Check sheet for the modelled part. Datum: model origin and axes. Units: mm. Face numbers are marked on the shaded views. A direction names the side the tool comes from. Round coordinates to 2 decimals unless told otherwise and drop trailing zeros. Order: outer loops, then holes, each group sorted by start corner. A loop starts at its lowest first (then second) coordinate and runs counter-clockwise, first axis right, second up.
(1) Tool access check on the marked faces 1 and 2. Record the directions out of +Z, -Z, +X, -X, +Y, -Y that give a thin tool (end or side, any length) a straight path to the whole face; none if there is none.
(2) Thickness scan on probe 1 along X at (y, z) = (20.5, 232.5); probe 2 along X at (y, z) = (-2.5, 214.5). Record the ranges inside material, lowest first.
(3) Depth check by flat-ended pin: pin 1 (13 mm diameter, centred on x = 7, z = 259.5, fed in from +Y); pin 2 (2 mm diameter, centred on x = -1, z = 291.5, fed in from +Y); pin 3 (1.5 mm diameter, centred on y = 13.5, z = 130, fed in from +X). Enter the tip coordinate at first touch or a pass-through.
(4) Sectioned sample at A-A, the plane z = 321. Enter the section's corners in (x, y).
(5) Sectioned sample at B-B, the plane x = 10. Enter the section's corners in (y, z), and give its area (3 significant figures).
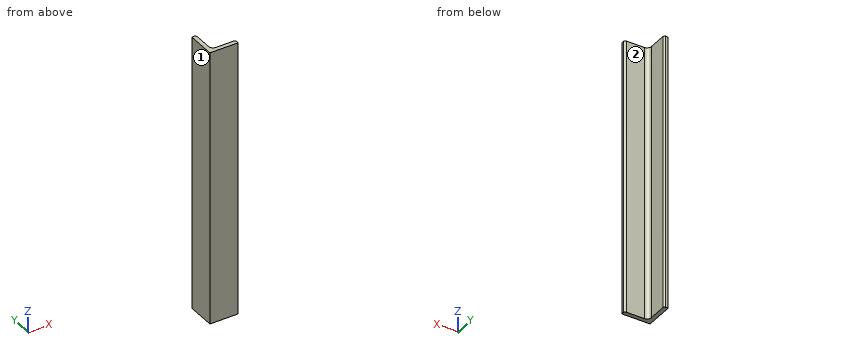
Autodesk Inventor part; units mm, degrees
ref_plane "Start Plane" through (0, 0, 0) normal (0, 0, 1) x (1, 0, 0)
ref_plane "End Plane" through (0, 0, 390) normal (0, 0, 1) x (1, 0, 0)
ref_plane "YZ Plane" through (0, 0, 0) normal (1, 0, 0) x (0, 1, 0)
ref_plane "Start Plane" through (0, 0, 0) normal (0, 0, 1) x (1, 0, 0)
ref_plane "End Plane" through (0, 0, 390) normal (0, 0, 1) x (1, 0, 0)
sketch "Sketch" plane through (0, 0, 0) normal (0, 0, 1) x (1, 0, 0)
  line L0 (-5.9502, 0.0498) -> (-5.9502, 25.6498)
  line L1 (-11.9502, 28.0498) -> (-8.3502, 28.0498)
  line L2 (-11.9502, -11.9502) -> (-11.9502, 28.0498)
  line L3 (-11.9502, -11.9502) -> (28.0498, -11.9502)
  line L4 (28.0498, -8.3502) -> (28.0498, -11.9502)
  line L5 (0.0498, -5.9502) -> (25.6498, -5.9502)
  arc A0 (-5.9502, 0.0498) -> (0.0498, -5.9502) centre (0.0498, 0.0498) ccw
  arc A1 (-5.9502, 25.6498) -> (-8.3502, 28.0498) centre (-8.3502, 25.6498) ccw
  arc A2 (28.0498, -8.3502) -> (25.6498, -5.9502) centre (25.6498, -8.3502) ccw
  line L6 (0, 36.6463) -> (0, -20.0496) construction
  line L7 (-20.0496, 0) -> (36.6463, 0) construction
  point P0 (-5.9502, -5.9502)
  point P1 (-5.9502, 28.0498)
  point P2 (28.0498, -5.9502)
  dimension "d4" = 40
  dimension "d6" = 40
  dimension "d8" = 6
  dimension "d10" = 6
  dimension "d17" = 6
  dimension "d18" = 2.4
  dimension "d19" = 11.9502
  dimension "d20" = 11.9502
extrude "Body" add sketch "Sketch" along normal up to surface (390 mm away) from surface at 0
sketch "Sketch3" plane through (0, 0, 0) normal (0, 0, 1) x (1, 0, 0)
  line L0 (0, 0) -> (10, 0)
ref_plane "Work Plane10" through (0, 0, 0) normal (0, -1, 0) x (1, 0, 0)
sketch "Sketch4" plane through (0, 0, 0) normal (0, -1, 0) x (1, 0, 0)
  line L0 (-2, 0) -> (12, 0)
  line L1 (-2, 390) -> (12, 390)
  dimension "d24" = 390
equation "\"d4\" = b"
equation "\"d6\" = b"
equation "\"d17\" = R"
equation "\"d18\" = R1"
equation "\"d19\" = ex"
equation "\"d20\" = d19"
equation "\"d11\" = G_L"
equation "\"b\" = 40"
equation "\"ParT\" = 6"
equation "\"R\" = 6"
equation "\"R1\" = 2.4"
equation "\"G_L\" = d24"
equation "\"G_OFFSET_START\" = 0"
equation "\"G_OFFSET_END\" = 0"
properties part number "BS 4848 - 40x40x6-390" material "Steel, Mild"
Derived:
1. face 1: +Z, -Z, -X, +Y, -Y
1. face 2: +Z, -Z, +X, +Y
2. probe 1: x = -11.95 to -5.95
2. probe 2: x = -11.95 to -5.38
3. pin 1: stops at y = -5.95
3. pin 2: stops at y = -5.59
3. pin 3: stops at x = -5.95
4. outline: (-11.95, -11.95) - (28.05, -11.95) - (28.05, -8.35) arc R2.4 ccw to (25.65, -5.95) - (0.05, -5.95) arc R6 cw to (-5.95, 0.05) - (-5.95, 25.65) arc R2.4 ccw to (-8.35, 28.05) - (-11.95, 28.05) - close
5. outline: (-11.95, 0) - (-5.95, 0) - (-5.95, 390) - (-11.95, 390) - close
5. area: 2,340 mm2
